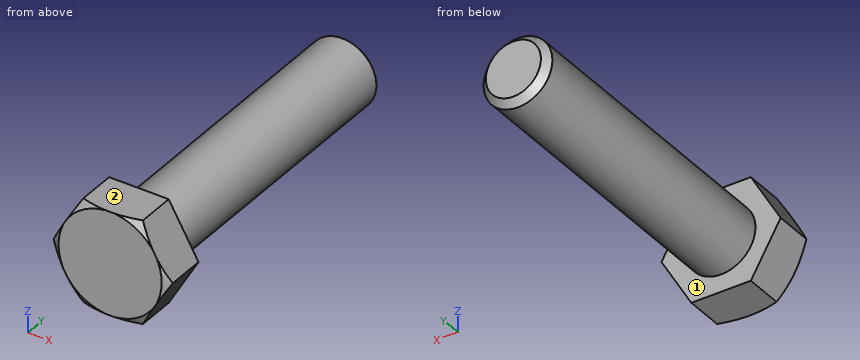
```python
from build123d import *

# Parameters (mm, degrees)
EXTRUDE_1_DEPTH = 12.5
SKETCH_2_R      = 10
EXTRUDE_2_DEPTH = 90
CHAMFER_1_SIZE  = 2


with BuildPart() as part:
    # 草图1 → 凸台-拉伸1 (new body)
    with BuildSketch(Plane(origin=(0, 0, 0), x_dir=(1, 0, 0), z_dir=(0, 1, 0))):
        Polygon((8.660254038, -15), (17.320508076, 0), (8.660254038, 15), (-8.660254038, 15), (-17.320508076, 0), (-8.660254038, -15), align=None)
    extrude(amount=EXTRUDE_1_DEPTH)

    # 草图2 → 凸台-拉伸2 (add)
    with BuildSketch(Plane(origin=(0, 12.5, 0), x_dir=(1, 0, 0), z_dir=(0, 1, 0))):
        with Locations(Location((0, 0, 0), (0, 0, 90))):
            Circle(SKETCH_2_R)
    extrude(amount=EXTRUDE_2_DEPTH)

    # 倒角1
    chamfer_1_edges = [part.edges().sort_by_distance(p)[0] for p in [
        (0, 102.5, 10),
    ]]
    chamfer(chamfer_1_edges, length=CHAMFER_1_SIZE)

    # 草图3 → 切除-旋转3 (revolve, cut)
    with BuildSketch(Plane(origin=(8.660254038, 0, 0), x_dir=(1, 0, 0), z_dir=(0, 0, 1))):
        Polygon((-23.660254038, 0), (-25.980762114, 1.339745962), (-25.980762114, 0), align=None)
    revolve(axis=Axis((0, 0, 0), (0, 1, 0)), mode=Mode.SUBTRACT)


solid = part.part
```
The listing builds one solid part. Answer for the finished solid, in the listing's coordinates (mm). Face numbers are marked on the shaded views. A direction names the side the tool comes from. Give positions to 0.01 mm unless a question says otherwise; leave off trailing zeros. Loops run counter-clockwise (first coordinate to the right, second up) from the corner with the lowest first, then second, coordinate; pieces in that order, holes last. Notation, with made-up numbers: (34.25, 14.25) - (67.25, 14.25) arc R10 ccw to (67.25, 33.25) - close; hole circle Ø2 at (6.5, -29.5). An arc over 180 degrees is marked (long way). Answer as CSV lines item,"result". Start each with the question number.
Item 1: Find the intervals of material crossed by line 1 (Y direction, x = 10.5, z = 10); line 2 (X direction, y = 68, z = -0.5); line 3 (Z direction, x = 3, y = 73.5), in increasing order. Write a range as from..to.
Item 2: Each of these flat-tipped pins is pushed along its axis until it touches: pin 1 (3 mm diameter, centred on x = 7.5, z = 10, fed in from -Y); pin 2 (2 mm diameter, centred on y = 63, z = 7.5, fed in from +X); pin 3 (10 mm diameter, centred on x = 13.5, y = 34, fed in from -Z); pin 4 (4 mm diameter, centred on y = 13.5, z = -9, fed in from +X). Where does it stop, or does it pass through?
Item 3: A cutting plane is placed at A-A on y = 88. Determine the outline of the cut face in (x, z), then the cut area to 3 significant figures.
Item 4: For the marked faces 1 and 2, determine the directions among +Z, -Z, +X, -X, +Y, -Y from which every point of the face is accessible in a straight line to the end or side of a thin tool.
Found:
1,line 1,"y = 0..12.5"
1,line 2,"x = -9.99..9.99"
1,line 3,"z = -9.54..9.54"
2,pin 1,"stops at y = 0"
2,pin 2,"stops at x = 7.6"
2,pin 3,"stops at z = -5.27"
2,pin 4,"stops at x = 13.12"
3,outline,"circle Ø20 at (0, 0)"
3,area,"314 mm^2"
4,face 1,"+Y"
4,face 2,"+Z, +X, -X, +Y, -Y"
